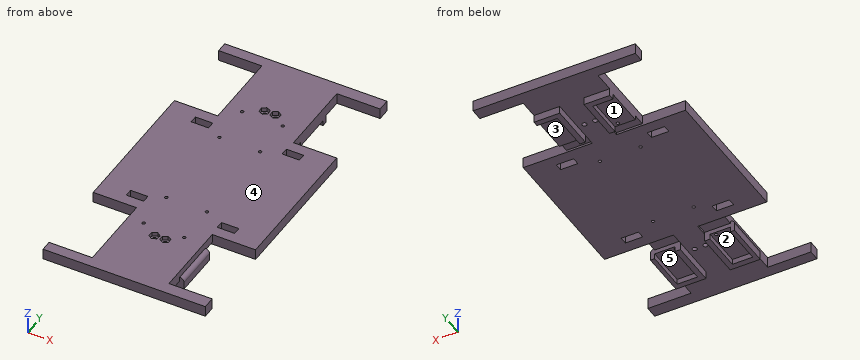
```python
from build123d import *

# Parameters (mm, degrees)
BOSS_EXTRUDE1_DEPTH       = 10
BOSS_EXTRUDE3_DEPTH       = 7
SKETCH4_W                 = 18.8
SKETCH4_H                 = 48.722574615
SKETCH4_H_2               = 48.326634129
BOSS_EXTRUDE4_DEPTH       = 2
CUT_EXTRUDE2_DEPTH        = 9
SKETCH7_R                 = 2.165
CUT_EXTRUDE3_DEPTH        = 336.559234711
CUT_EXTRUDE4_DEPTH        = 3.8
BOSS_EXTRUDE5_DEPTH       = 42.245940515
SKETCH10_W                = 40
SKETCH10_H                = 8.663840555
SKETCH10_H_2              = 10
CUT_EXTRUDE5_DEPTH        = 336.559234711
SKETCH11_W                = 40
SKETCH11_H                = 17.043549312
BOSS_EXTRUDE6_DEPTH       = 10
CUT_EXTRUDE6_REACH        = 337.841
SKETCH12_W                = 16
SKETCH12_H                = 7
F_1_5MM_DOWEL_HOLE1_D     = 2.85
F_1_5MM_DOWEL_HOLE1_DEPTH = 12


with BuildPart() as part:
    # Sketch2 → Boss-Extrude1 (new body)
    with BuildSketch(Plane.XY):
        Polygon((0, 0), (-150, 0), (-150, 20), (-110, 20), (-110, 100), (-150, 100), (-150, 200), (-110, 200), (-110, 280), (-150, 280), (-150, 300), (0, 300), (0, 280), (-40, 280), (-40, 200), (0, 200), (0, 100), (-40, 100), (-40, 20), (0, 20), align=None)
    extrude(amount=BOSS_EXTRUDE1_DEPTH)

    # Sketch3 → Boss-Extrude3 (add)
    with BuildSketch(Plane(origin=(0, 0, 0), x_dir=(-1, 0, 0), z_dir=(0, 0, -1))):
        Polygon((40, 34.233876073), (58.8, 34.233876073), (58.8, 82.956450688), (63.8, 82.956450688), (63.8, 29.233876073), (40, 29.233876073), align=None)
        Polygon((110, 34.629816559), (91.2, 34.629816559), (91.2, 82.956450688), (86.2, 82.956450688), (86.2, 29.233876073), (110, 29.233876073), align=None)
    boss_extrude3 = extrude(amount=BOSS_EXTRUDE3_DEPTH)

    # Sketch4 → Boss-Extrude4 (add)
    with BuildSketch(Plane(origin=(0, 0, 0), x_dir=(-1, 0, 0), z_dir=(0, 0, -1))):
        with Locations((49.4, 58.595163381)):
            Rectangle(SKETCH4_W, SKETCH4_H)
        with Locations((100.6, 58.793133624)):
            Rectangle(SKETCH4_W, SKETCH4_H_2)
    boss_extrude4 = extrude(amount=BOSS_EXTRUDE4_DEPTH)

    # Sketch6 → Cut-Extrude2 (cut)
    with BuildSketch(Plane(origin=(0, 0, -7), x_dir=(-1, 0, 0), z_dir=(0, 0, -1))):
        Polygon((40, 82.956450688), (55.172474276, 82.956450688), (63.8, 82.956450688), (63.8, 71.479816588), (58.8, 71.479816588), (40, 71.479816588), align=None)
        Polygon((91.2, 82.956450688), (110, 82.956450688), (110, 71.479816588), (95.490694749, 71.479816588), (86.2, 71.479816588), (86.2, 82.956450688), align=None)
    cut_extrude2 = extrude(amount=-CUT_EXTRUDE2_DEPTH, mode=Mode.SUBTRACT)

    # Sketch7 → Cut-Extrude3 (cut, through all)
    with BuildSketch(Plane(origin=(0, 0, 0), x_dir=(-1, 0, 0), z_dir=(0, 0, -1))):
        with Locations((70, 59.0298166)):
            Circle(SKETCH7_R)
        with Locations((80, 59.0298166)):
            Circle(SKETCH7_R)
    cut_extrude3 = extrude(amount=-CUT_EXTRUDE3_DEPTH, mode=Mode.SUBTRACT)

    # Sketch8 → Cut-Extrude4 (cut)
    with BuildSketch(Plane.XY.offset(10)):
        Polygon((-83.740057918, 61.707869394), (-84.189290711, 57.129857828), (-80.449232793, 54.451805034), (-76.259942082, 56.351763806), (-75.810709289, 60.929775372), (-79.550767207, 63.607828166), align=None)
        Polygon((-70, 63.6298166), (-73.983716857, 61.3298166), (-73.983716857, 56.7298166), (-70, 54.4298166), (-66.016283143, 56.7298166), (-66.016283143, 61.3298166), align=None)
    cut_extrude4 = extrude(amount=-CUT_EXTRUDE4_DEPTH, mode=Mode.SUBTRACT)

    # Sketch9 → Boss-Extrude5 (add)
    with BuildSketch(Plane.XZ.offset(-29.233876073)):
        with BuildLine():
            Line((-110, -7), (-113.9, -7))
            Line((-113.9, -7), (-113.9, 0))
            ThreePointArc((-113.9, 0), (-112.757716447, 2.757716447), (-110, 3.9))
            Line((-110, 3.9), (-110, 0))
            Line((-110, 0), (-110, -7))
        make_face()
        with BuildLine():
            Line((-40, -7), (-36.1, -7))
            Line((-36.1, -7), (-36.1, 0))
            ThreePointArc((-36.1, 0), (-37.242283553, 2.757716447), (-40, 3.9))
            Line((-40, 3.9), (-40, 0))
            Line((-40, 0), (-40, -7))
        make_face()
    extrude(amount=-BOSS_EXTRUDE5_DEPTH)

    # Mirror2: Boss-Extrude3, Boss-Extrude4, Cut-Extrude2 across plane
    add(boss_extrude3.mirror(Plane.ZX.offset(150)))
    add(boss_extrude4.mirror(Plane.ZX.offset(150)))
    add(cut_extrude2.mirror(Plane.ZX.offset(150)), mode=Mode.SUBTRACT)

    # Mirror3: Cut-Extrude3 across plane
    add(cut_extrude3.mirror(Plane.ZX.offset(150)), mode=Mode.SUBTRACT)

    # Mirror4: Cut-Extrude4 across plane
    add(cut_extrude4.mirror(Plane.ZX.offset(150)), mode=Mode.SUBTRACT)

    # Sketch10 → Cut-Extrude5 (cut, through all)
    with BuildSketch(Plane(origin=(0, 0, 0), x_dir=(-1, 0, 0), z_dir=(0, 0, -1))):
        with Locations((20, 284.331920277)):
            Rectangle(SKETCH10_W, SKETCH10_H)
        with Locations((130, 285)):
            Rectangle(SKETCH10_W, SKETCH10_H_2)
    cut_extrude5 = extrude(amount=-CUT_EXTRUDE5_DEPTH, mode=Mode.SUBTRACT)

    # Mirror5: Cut-Extrude5 across plane
    add(cut_extrude5.mirror(Plane.ZX.offset(150)), mode=Mode.SUBTRACT)

    # Sketch11 → Boss-Extrude6 (add, through all)
    with BuildSketch(Plane(origin=(0, 0, 0), x_dir=(-1, 0, 0), z_dir=(0, 0, -1))):
        with Locations((20, 208.521774656)):
            Rectangle(SKETCH11_W, SKETCH11_H)
        with Locations((130, 208.521774656)):
            Rectangle(SKETCH11_W, SKETCH11_H)
    boss_extrude6 = extrude(amount=-BOSS_EXTRUDE6_DEPTH)

    # Mirror6: Boss-Extrude6 across plane
    add(boss_extrude6.mirror(Plane.ZX.offset(150)))

    # Sketch12 → Cut-Extrude6 (cut, up to next)
    with BuildSketch(Plane.XY.offset(10), mode=Mode.PRIVATE) as cut_extrude6_sk1:
        with Locations((-117, 203.543549312)):
            Rectangle(SKETCH12_W, SKETCH12_H)
    cut_extrude6_tool1 = extrude(cut_extrude6_sk1.sketch, amount=-CUT_EXTRUDE6_REACH, mode=Mode.PRIVATE) & part.part
    # Sketch12 → Cut-Extrude6 (cut, up to next)
    with BuildSketch(Plane.XY.offset(10), mode=Mode.PRIVATE) as cut_extrude6_sk2:
        with Locations((-33, 203.543549312)):
            Rectangle(SKETCH12_W, SKETCH12_H)
    cut_extrude6_tool2 = extrude(cut_extrude6_sk2.sketch, amount=-CUT_EXTRUDE6_REACH, mode=Mode.PRIVATE) & part.part
    # Sketch12 → Cut-Extrude6 (cut, up to next)
    with BuildSketch(Plane.XY.offset(10), mode=Mode.PRIVATE) as cut_extrude6_sk3:
        with Locations((-117, 96.456450688)):
            Rectangle(SKETCH12_W, SKETCH12_H)
    cut_extrude6_tool3 = extrude(cut_extrude6_sk3.sketch, amount=-CUT_EXTRUDE6_REACH, mode=Mode.PRIVATE) & part.part
    # Sketch12 → Cut-Extrude6 (cut, up to next)
    with BuildSketch(Plane.XY.offset(10), mode=Mode.PRIVATE) as cut_extrude6_sk4:
        with Locations((-33, 96.456450688)):
            Rectangle(SKETCH12_W, SKETCH12_H)
    cut_extrude6_tool4 = extrude(cut_extrude6_sk4.sketch, amount=-CUT_EXTRUDE6_REACH, mode=Mode.PRIVATE) & part.part
    add(cut_extrude6_tool1.solids().sort_by_distance((-117, 203.543549, 10))[0], mode=Mode.SUBTRACT)
    add(cut_extrude6_tool2.solids().sort_by_distance((-33, 203.543549, 10))[0], mode=Mode.SUBTRACT)
    add(cut_extrude6_tool3.solids().sort_by_distance((-117, 96.456451, 10))[0], mode=Mode.SUBTRACT)
    add(cut_extrude6_tool4.solids().sort_by_distance((-33, 96.456451, 10))[0], mode=Mode.SUBTRACT)

    # Ø1.5mm Dowel Hole1
    with Locations(Plane.XY.offset(10)):
        with Locations((-57.884566311, 231.352487628), (-95.402442942, 231.352487628), (-95.402442942, 193.834610997), (-57.884566311, 193.834610997), (-95.402442942, 68.647512372), (-57.884566311, 106.165389003), (-57.884566311, 68.647512372), (-95.402442942, 106.165389003)):
            Hole(F_1_5MM_DOWEL_HOLE1_D / 2, depth=F_1_5MM_DOWEL_HOLE1_DEPTH)


solid = part.part
```
Source: CAD feature listing. Evaluate the final solid. Frame: model axes, mm. Face numbers are marked on the shaded views. A direction names the side the tool comes from. Round coordinates to 2 decimals unless told otherwise and drop trailing zeros. Order: outer loops, then holes, each group sorted by start corner. A loop starts at its lowest first (then second) coordinate and runs counter-clockwise, first axis right, second up. Notation, with made-up numbers: (83.25, 71) -> (123.25, 71) arc R20 cw to (123.25, 78) -> close; hole circle Ø8 at (-39, 11). An arc over 180 degrees is marked (long way). Use CSV: the item, a comma, the result in double quotes.
(1) Ray query, L1, parallel to X at y = 231, z = 2.25; L2, parallel to Y at x = -140, z = 0.25; L3, parallel to Y at x = -80, z = 1.75. Return the intervals inside material, ascending.
Report:
L1,"-110 to -96.78, -94.02 to -59.27, -56.5 to -40"
L2,"0 to 10, 82.96 to 217.04, 290 to 300"
L3,"0 to 56.86, 61.19 to 238.81, 243.14 to 300"
(2) Pull-direction query (Y, two-part tool) for the marked faces 4 and 5; classes: +Y half, -Y half, draft (parallel to the pull), parting line (faces both ways), or undercut.
Report:
face 4,"draft"
face 5,"undercut"
(3) Section A-A on x = -102. Return the cut outline in (y, z).
Report:
outline,"(0, 0) -> (29.23, 0) -> (29.23, -7) -> (34.63, -7) -> (34.63, -2) -> (71.48, -2) -> (71.48, 2) -> (82.96, 2) -> (82.96, 0) -> (217.04, 0) -> (217.04, 2) -> (228.52, 2) -> (228.52, -2) -> (265.37, -2) -> (265.37, -7) -> (270.77, -7) -> (270.77, 0) -> (300, 0) -> (300, 10) -> (0, 10) -> close"
(4) Access query for the marked faces 1, 2 and 3. Directions: +Z, -Z, +X, -X, +Y, -Y. A direction counts if a zero-diameter tool reaches every point of the face in a straight line with its end or side. Return the directions, or none.
Report:
face 1,"-Z, -X"
face 2,"-Z"
face 3,"-Z, +X"
(5) First-contact query: pin 1 Ø3.5 at (x, y) = (-57.88, 106.17) entering from +Z; pin 2 Ø5.5 at (y, z) = (48, -3.5) entering from -X; pin 3 Ø0.6 at (y, z) = (76, 1) entering from -X; pin 4 Ø5 at (y, z) = (34, 4.5) entering from +X. Flat tips, straight axial feed; report the tip coordinate or a pass-through.
Report:
pin 1,"z = 10"
pin 2,"x = -113.9"
pin 3,"x = -86.2"
pin 4,"x = -36.65"
(6) Section B-B on y = 20.5. Return the cut outline in (x, z), and give its area (3 significant figures).
Report:
outline,"(-110, 0) -> (-40, 0) -> (-40, 10) -> (-110, 10) -> close"
area,"700 mm^2"
